```python
from build123d import *

# Parameters (mm, degrees)
F0_R     = 1.5694812218
F1_DEPTH = 50.8


# Not quite as in the source:
# - a feature names something its author has since deleted; it is built from what else it names


with BuildPart() as f1:
    # F0 (on Front) → F1 (new body)
    with BuildSketch(Plane.XZ):
        Polygon((6.6879468774, 24.9597575449), (-6.6879468774, 24.9597575449), (-18.2718106675, 18.2718106675), (-24.9597575449, 6.6879468774), (-24.9597575449, -6.6879468774), (-18.2718106675, -18.2718106675), (-6.6879468774, -24.9597575449), (6.6879468774, -24.9597575449), (18.2718106675, -18.2718106675), (24.9597575449, -6.6879468774), (24.9597575449, 6.6879468774), (18.2718106675, 18.2718106675), align=None)
        Circle(F0_R, mode=Mode.SUBTRACT)
    extrude(amount=F1_DEPTH)


solid = f1.part
```
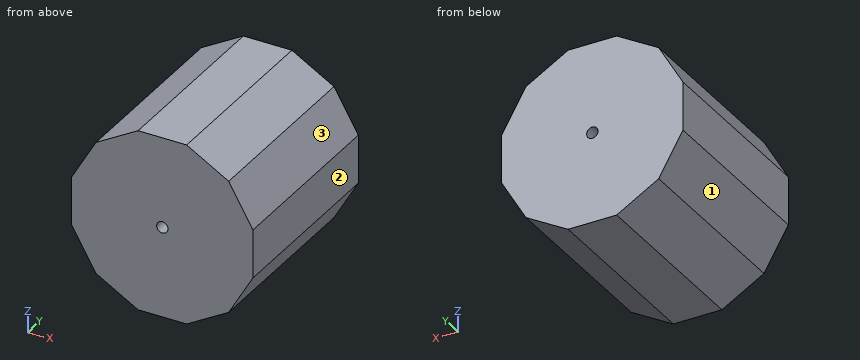
Part model, mm, in its own coordinate system. Face numbers are marked on the shaded views. Give positions to 0.01 mm unless a question says otherwise; leave off trailing zeros. Write each loop counter-clockwise with the first axis right and the second up, starting at its lowest first coordinate (ties: lowest second). Pieces come first, ordered by that corner, then holes. Notation, with made-up numbers: M 6,-34.5 L 50,-34.5 A20 ccw 50,-18.5 Z; hole C 7,7 d7. An arc over 180 degrees is marked long. Use CSV: the item, a comma, the result in double quotes.
Item 1: Drill centre lines: probe 1 along Z at (x, y) = (0, -33); probe 2 along X at (y, z) = (-9, -12.5); probe 3 along Z at (x, y) = (-10, -30). Where is each one in solid material? Low to high.
Taken from the geometry:
probe 1,"z = -24.96 to -1.57, 1.57 to 24.96"
probe 2,"x = -21.6 to 21.6"
probe 3,"z = -23.05 to 23.05"
Item 2: Slice it at A-A on z = 0. Write the cut outline in (x, y).
Taken from the geometry:
outline,"M -24.96,-50.8 L -1.57,-50.8 L -1.57,0 L -24.96,0 Z; M 1.57,-50.8 L 24.96,-50.8 L 24.96,0 L 1.57,0 Z"
Item 3: Slice it at C-C on x = 0. Write the cut outline in (y, z).
Taken from the geometry:
outline,"M -50.8,-24.96 L 0,-24.96 L 0,-1.57 L -50.8,-1.57 Z; M -50.8,1.57 L 0,1.57 L 0,24.96 L -50.8,24.96 Z"
Item 4: Pull direction Z, two halves, no side cores. Call the marked faces 1, 2 and 3: +Z half, -Z half, draft (parallel to the pull), parting line (faces both ways), or undercut.
Taken from the geometry:
face 1,"-Z half"
face 2,"draft"
face 3,"+Z half"
Item 5: Pin check, flat tips, straight feed: P1, Ø3, axis at y = -29, z = -10.5, coming from the -X side; P2, Ø1, axis at y = -24, z = -20, coming from the -X side; P3, Ø1.5, axis at y = -44.5, z = -15, coming from the -X side. Stop position of each tip, or through.
Taken from the geometry:
P1,"stops at x = -23.62"
P2,"stops at x = -16.14"
P3,"stops at x = -20.59"
Item 6: Slice it at B-B on y = -11. Write the cut outline in (x, z), plus the area to 3 significant figures.
Taken from the geometry:
outline,"M -24.96,-6.69 L -18.27,-18.27 L -6.69,-24.96 L 6.69,-24.96 L 18.27,-18.27 L 24.96,-6.69 L 24.96,6.69 L 18.27,18.27 L 6.69,24.96 L -6.69,24.96 L -18.27,18.27 L -24.96,6.69 Z; hole C 0,0 d3.14"
area,"2,000 mm²"
Item 7: Slice it at D-D on x = -13. Write the cut outline in (y, z), plus the area to 3 significant figures.
Taken from the geometry:
outline,"M -50.8,-21.32 L 0,-21.32 L 0,21.32 L -50.8,21.32 Z"
area,"2,170 mm²"
